from build123d import *

# Parameters (mm, degrees)
SKETCH1_R           = 2.159
SKETCH1_R_2         = 4.7625
BOSS_EXTRUDE1_DEPTH = 2.9718
SKETCH2_R           = 1.524
CUT_EXTRUDE2_DEPTH  = 3.9718


with BuildPart() as part:
    # Sketch1 → Boss-Extrude1 (new body)
    with BuildSketch(Plane.XY):
        Polygon((-109.126324886, 41.028491651), (-109.126324886, 15.481473491), (-106.848322687, 23.983093437), (-103.977784316, 23.213934999), (-106.443035721, 14.013491503), (-54.143973439, 0), (-25.4, 0), (-25.4, 2.9718), (-12.7, 2.9718), (-12.7, 0), (0, 0), (0, 6.35), (2.9718, 6.35), (2.9718, 19.05), (0, 19.05), (0, 25.4), (-23.123469124, 27.310236218), (-25.4, 25.4), (-33.563402643, 35.128764428), (-31.286871767, 37.039000646), (-39.45027441, 46.767765074), (-41.726805286, 44.857528855), (-49.890207929, 54.586293283), (-47.613677053, 56.496529501), (-51.67877148, 61.341120389), (-83.931779224, 34.277633487), align=None)
        with Locations((-73.773359536, 10.321661037)):
            Circle(SKETCH1_R, mode=Mode.SUBTRACT)
        with Locations((-90.888775854, 22.993747625)):
            Circle(SKETCH1_R_2, mode=Mode.SUBTRACT)
        with Locations((-69.730347232, 25.410388369)):
            Circle(SKETCH1_R, mode=Mode.SUBTRACT)
    extrude(amount=BOSS_EXTRUDE1_DEPTH)

    # Sketch2 → Cut-Extrude2 (cut, through all)
    with BuildSketch(Plane.XY.offset(2.9718)):
        with Locations((1.4859, 12.7)):
            Circle(SKETCH2_R)
        with Locations((-6.35, 1.4859)):
            Circle(SKETCH2_R)
        with Locations((-102.61910191, 34.025683513)):
            Circle(SKETCH2_R)
        Polygon((-22.225, 15.6718), (-15.875, 15.6718), (-15.875, 13.1318), (-17.526, 13.1318), (-17.526, 2.9718), (-20.574, 2.9718), (-20.574, 13.1318), (-22.225, 13.1318), align=None)
        Polygon((-57.578121696, 43.990699533), (-53.496420374, 39.126317319), (-51.550667489, 40.758997848), (-52.611909832, 42.023737223), (-44.82889829, 48.554459338), (-46.788114925, 50.8893628), (-54.571126467, 44.358640686), (-55.63236881, 45.623380062), align=None)
    extrude(amount=-CUT_EXTRUDE2_DEPTH, mode=Mode.SUBTRACT)


solid = part.part
Verification items for the finished model (mm, model axes). A direction names the side the tool comes from. Coordinates: 2 decimals unless noted, no trailing zeros. Order: outer loops, then holes, each group sorted by start corner. A loop starts at its lowest first (then second) coordinate and runs counter-clockwise, first axis right, second up. Notation, with made-up numbers: M -12.75,51 L -4.75,51 A21 ccw -4.75,87 Z; hole C -1,37.5 d6. An arc over 180 degrees is marked long. One line per item, written item: value. Start each with the question number.
Item 1: Sectioned sample at C-C (y = 31). Enter the section's corners in (x, z).
Item 2: Sectioned sample at B-B (z = 1.95). Count the separate pieces of the cut face and the enclosed holes in it, then the cut area to 3 significant figures.
Item 3: Mould release check, pull along X, two halves, no side actions. Record for faces 5 (the flat face through (2.972, 16, 1)), 6 (the flat face through (-20.574, 8, 2)), 7 (the flat face through (-108.003, 19.673, 1.465)), 8 (the flat face through (-80.66, 7.105, 1.465)): released by +X, released by -X, zero draft, split by the parting line, or undercut.
Item 4: Sectioned sample at A-A (y = 21). Enter the section's corners in (x, z).
Item 5: Gauge pin test, flat ends, axial feed: pin 1 (0.8 mm diameter, centred on x = -21.5, z = 1.5, fed in from +Y); pin 2 (1.8 mm diameter, centred on x = -6.35, y = 1.49, fed in from -Z); pin 3 (0.9 mm diameter, centred on y = 4.5, z = 2, fed in from +X); pin 4 (0.9 mm diameter, centred on x = 1.5, z = 1, fed in from +Y). Record the tip position at first contact, or that the pin passes through.
Item 6: Scan lines: probe 1 along X at (y, z) = (24.5, 0.7); probe 2 along X at (y, z) = (21, 1.9); probe 3 along Y at (x, z) = (-38.5, 1.4). Record each from-to range of solid material in increasing order.
Item 7: Access from +Z, -Z, +X, -X, +Y, -Y to the whole of each face (thin tool, end or side, straight path). Record for faces 1 (the flat face through (0, 22, 1)), 2 (the flat face through (-32.44, 36.07, 1.47)), 3 (the flat face through (0, 3, 1)), 4 (the flat face through (-19, 15.672, 2)).
Item 8: Sectioned sample at D-D (x = -10). Enter the section's corners in (y, z), then the cut area to 3 significant figures.
Conclusion:
1. outline: M -109.13,0 L -30.1,0 L -30.1,2.97 L -109.13,2.97 Z
2. separate pieces: 1
2. enclosed holes: 4
2. area: 3,640 mm^2
3. face 5: released by +X
3. face 6: undercut
3. face 7: undercut
3. face 8: released by -X
4. outline: M -109.13,0 L -107.65,0 L -107.65,2.97 L -109.13,2.97 Z; M -104.57,0 L -95.21,0 L -95.21,2.97 L -104.57,2.97 Z; M -86.56,0 L 0,0 L 0,2.97 L -86.56,2.97 Z
5. pin 1: stops at y = 27.21
5. pin 2: passes through
5. pin 3: stops at x = 0
5. pin 4: stops at y = 19.05
6. probe 1: x = -109.13 to -95.41, -86.37 to -71.69, -67.77 to 0
6. probe 2: x = -109.13 to -107.65, -104.57 to -95.21, -86.56 to 0
6. probe 3: y = 0 to 45.64
7. face 1: +Z, -Z, +X, +Y
7. face 2: +Z, -Z, +X
7. face 3: +Z, -Z, +X, -Y
7. face 4: +Z, -Z
8. outline: M 0,0 L 26.23,0 L 26.23,2.97 L 0,2.97 Z
8. area: 77.9 mm^2
